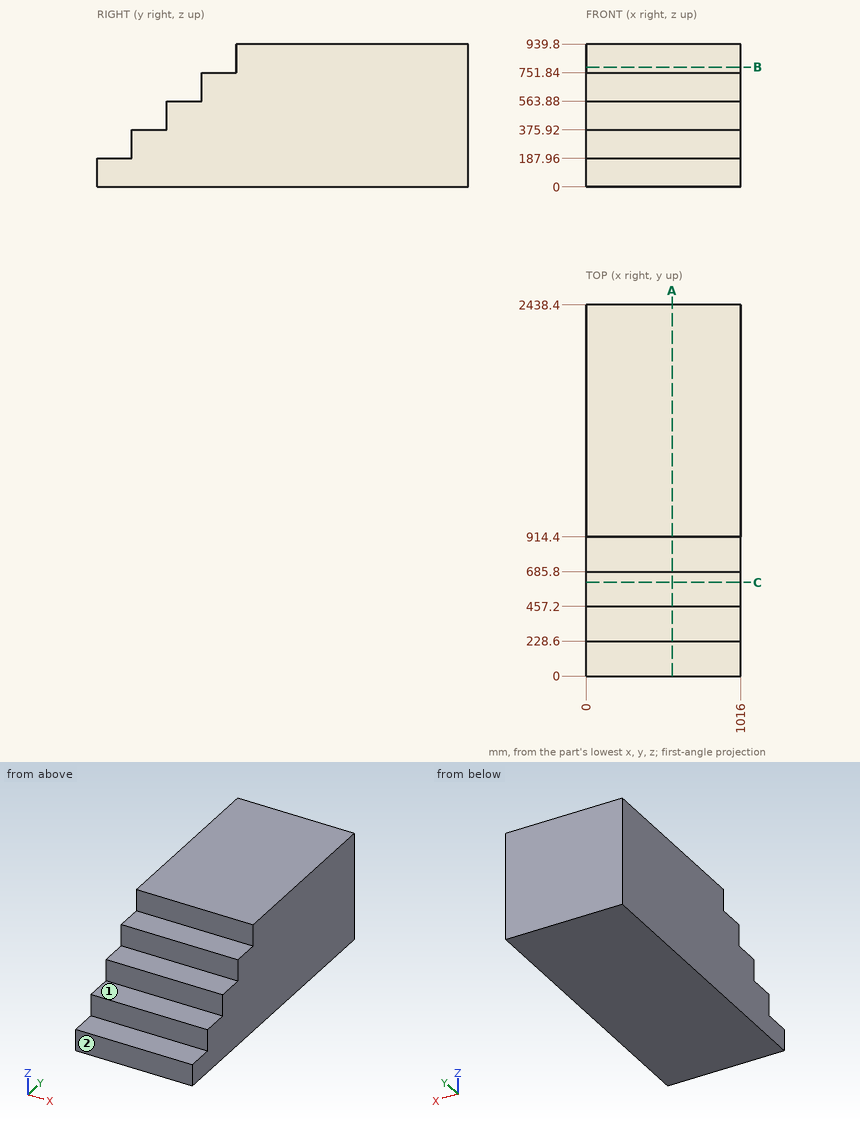
Could you check a few things on this drawing? It's one solid part, dimensions in mm from its lowest x, y, z. A direction names the side the tool comes from. Coordinates: 2 decimals unless noted, no trailing zeros. Order: outer loops, then holes, each group sorted by start corner. A loop starts at its lowest first (then second) coordinate and runs counter-clockwise, first axis right, second up.
1) Will these pins go through, and if not, where does the flat tip stop? pin 1 (1.5 mm diameter, centred on x = 426.5, y = 1493.5, fed in from -Z); pin 2 (12 mm diameter, centred on x = 305, z = 448.5, fed in from -Y); pin 3 (10 mm diameter, centred on x = 284, y = 340, fed in from +Z); pin 4 (10 mm diameter, centred on x = 390, z = 689, fed in from -Y).
2) Imagine slicing it at A-A on x = 564. List the corners of the cut face in (y, z) for me.
3) I need wall thicknesses on line 1 (Z direction, x = 552.5, y = 528); line 2 (Z direction, x = 848.5, y = 746); line 3 (Y direction, x = 548, z = 671.5). Which ranges of each line are inside material? Lowest first, please.
4) Which directions (+Z, -Z, +X, -X, +Y, -Y) give clear straight access to the entire face, cutting with the end or side of a thin tool? Please do the marked faces 1 and 2.
5) Imagine slicing it at B-B on z = 788.5. List the corners of the cut face in (x, y) for me.
6) Imagine slicing it at C-C on y = 615.5. List the corners of the cut face in (x, z) for me, and give its area (3 significant figures).
Response values:
1. pin 1: stops at z = 0
1. pin 2: stops at y = 457.2
1. pin 3: stops at z = 375.92
1. pin 4: stops at y = 685.8
2. outline: (0, 0) - (2438.4, 0) - (2438.4, 939.8) - (914.4, 939.8) - (914.4, 751.84) - (685.8, 751.84) - (685.8, 563.88) - (457.2, 563.88) - (457.2, 375.92) - (228.6, 375.92) - (228.6, 187.96) - (0, 187.96) - close
3. line 1: z = 0 to 563.88
3. line 2: z = 0 to 751.84
3. line 3: y = 685.8 to 2438.4
4. face 1: +Z, +X, -X, -Y
4. face 2: +Z, -Z, +X, -X, -Y
5. outline: (0, 914.4) - (1016, 914.4) - (1016, 2438.4) - (0, 2438.4) - close
6. outline: (0, 0) - (1016, 0) - (1016, 563.88) - (0, 563.88) - close
6. area: 573,000 mm2
